Work out the finished part from the listing and answer in its coordinate system (mm). Round coordinates to 2 decimals unless told otherwise and drop trailing zeros. Write each loop counter-clockwise with the first axis right and the second up, starting at its lowest first coordinate (ties: lowest second). Pieces come first, ordered by that corner, then holes.
1. A flat-ended cylindrical pin translates along its axis: pin 1 Ø4 at (x, z) = (-1, -37.5) entering from -Y. Find the tip coordinate at first contact, or state that the pin passes through.
2. Find section B-B (x = 10.16). Write down the section's boundary in (y, z), and give its area (3 significant figures).
3. Straight lines are drawn through the part: probe 1 along X at (y, z) = (2.9, 0); probe 2 along Z at (x, y) = (0, 3); probe 3 along X at (y, z) = (2.05, 1). For each, find the intervals that lie inside material, in ascending order.
4. Determine the mould class of faces 1 (the face through (4, 2, 5.055)), 2 (the face through (5.1, 1.628, -44.577)), 3 (the face through (8.586, 1.972, 0.207)) for opening direction Z: pulls with the +Z half, pulls with the -Z half, needs draft (parallel to the pull), parting line crosses it, or undercut.
5. Find section D-D (z = 0). Write down the section's boundary in (x, y), and give its area (3 significant figures).
6. Find section A-A (z = -14.5). Write down the section's boundary in (x, y).
7. Find section C-C (y = 0.55). Write down the section's boundary in (x, z) (3 decimals), and give its area (3 significant figures).
```python
from build123d import *

# Parameters (mm, degrees)
SKETCH1_R                      = 1.1303
BOSS_EXTRUDE1_DEPTH            = 3.302
F_4_CLEARANCE_HOLE1_AT_2_COUNT = 2
F_4_CLEARANCE_HOLE1_AT_2_PITCH = 10.16
SKETCH17_R                     = 6.35
CUT_EXTRUDE1_DEPTH             = 52.411789825
SKETCH18_R                     = 3.175
CUT_EXTRUDE2_DEPTH             = 52.411789825


with BuildPart() as part:
    # Sketch1 → Boss-Extrude1 (new body)
    with BuildSketch(Plane(origin=(0, 0, 0), x_dir=(1, 0, 0), z_dir=(0, 1, 0))):
        with BuildLine():
            Line((7.439072116, 42.978476899), (25.219072116, -1.573123101))
            ThreePointArc((25.219072116, -1.573123101), (24.962730525, -3.939424318), (22.86, -5.0546))
            Line((22.86, -5.0546), (-15.24, -5.0546))
            ThreePointArc((-15.24, -5.0546), (-17.37645185, -3.888344332), (-17.550975292, -1.460563379))
            Line((-17.550975292, -1.460563379), (2.769024708, 43.091036621))
            ThreePointArc((2.769024708, 43.091036621), (5.141202523, 44.576262541), (7.439072116, 42.978476899))
        make_face()
        with Locations(Location((0, 0, 0), (0, 0, 90))):
            Circle(SKETCH1_R, mode=Mode.SUBTRACT)
        with Locations(Location((10.16, 0, 0), (0, 0, 90))):
            Circle(SKETCH1_R, mode=Mode.SUBTRACT)
    extrude(amount=BOSS_EXTRUDE1_DEPTH)

    # Sketch16 → #4 Clearance Hole1 (revolve, cut)
    with BuildSketch(Plane(origin=(0, 0, 0), x_dir=(0, 0, -1), z_dir=(1, 0, 0))):
        Polygon((0, 0), (0, 3.302), (1.4732, 3.302), (1.4732, 2.103793743), (3.302, 0), align=None)
    f_4_clearance_hole1 = revolve(axis=Axis((0, -6.35, 0), (0, 1, 0)), mode=Mode.SUBTRACT)

    # #4 Clearance Hole1 at 2: #4 Clearance Hole1 ×2
    with Locations(*[(i * F_4_CLEARANCE_HOLE1_AT_2_PITCH, 0, 0) for i in range(1, F_4_CLEARANCE_HOLE1_AT_2_COUNT)]):
        add(f_4_clearance_hole1, mode=Mode.SUBTRACT)

    # Sketch17 → Cut-Extrude1 (cut, through all)
    with BuildSketch(Plane.XZ):
        with Locations(Location((5.08, -12.7, 0), (0, 0, 270))):
            Circle(SKETCH17_R)
    extrude(amount=-CUT_EXTRUDE1_DEPTH, mode=Mode.SUBTRACT)

    # Sketch18 → Cut-Extrude2 (cut, through all)
    with BuildSketch(Plane.XZ):
        with Locations(Location((5.08, -25.4, 0), (0, 0, 270))):
            Circle(SKETCH18_R)
    extrude(amount=-CUT_EXTRUDE2_DEPTH, mode=Mode.SUBTRACT)


solid = part.part
```
Worked answers:
1. pin 1: stops at y = 0
2. outline: (0, -36.16) - (3.3, -36.16) - (3.3, -16.51) - (0, -16.51) - close; (0, -8.89) - (3.3, -8.89) - (3.3, -1.47) - (2.1, -1.47) - (0, -3.3) - close; (0, 3.3) - (2.1, 1.47) - (3.3, 1.47) - (3.3, 5.05) - (0, 5.05) - close
2. area: 97.4 mm2
3. probe 1: x = -16.88 to -1.47, 1.47 to 8.69, 11.63 to 24.59
3. probe 2: z = -37.02 to -16.51, -8.89 to -1.47, 1.47 to 5.05
3. probe 3: x = -17.34 to -1.14, 1.14 to 9.02, 11.3 to 24.99
4. face 1: pulls with the +Z half
4. face 2: pulls with the -Z half
4. face 3: undercut
5. outline: (-16.88, 0) - (-3.3, 0) - (-1.47, 2.1) - (-1.47, 3.3) - (-16.88, 3.3) - close; (1.47, 2.1) - (3.3, 0) - (6.86, 0) - (8.69, 2.1) - (8.69, 3.3) - (1.47, 3.3) - close; (11.63, 2.1) - (13.46, 0) - (24.59, 0) - (24.59, 3.3) - (11.63, 3.3) - close
5. area: 110 mm2
6. outline: (-10.27, 0) - (-1.01, 0) - (-1.01, 3.3) - (-10.27, 3.3) - close; (11.17, 0) - (18.8, 0) - (18.8, 3.3) - (11.17, 3.3) - close
7. outline: (-17.551, 1.461) - (2.769, -43.091) arc R2.54 ccw to (7.439, -42.978) - (25.219, 1.573) arc R2.54 ccw to (22.86, 5.055) - (-15.24, 5.055) arc R2.54 ccw to start; hole circle Ø5.648 at (0, 0); hole circle Ø12.7 at (5.08, -12.7); hole circle Ø6.35 at (5.08, -25.4); hole circle Ø5.648 at (10.16, 0)
7. area: 1,000 mm2
